from build123d import *

# Parameters (mm, degrees)
AUFSATZ_LINEAR_AUSTRAGEN1_DEPTH = 2.5


with BuildPart() as part:
    # Skizze1 → Rotation1 (revolve)
    with BuildSketch(Plane.XY):
        with BuildLine():
            Line((0, 45), (0, 35))
            ThreePointArc((0, 35), (5, 40), (0, 45))
        make_face()
    revolve(axis=Axis((0, 0, 0), (0, 1, 0)))

    # Skizze2 → Aufsatz-Linear austragen1 (add, symmetric)
    with BuildSketch(Plane.XY):
        Polygon((0, 40), (-10, 5.773502692), (0, 0), (10, 5.773502692), align=None)
    extrude(amount=AUFSATZ_LINEAR_AUSTRAGEN1_DEPTH, both=True)


solid = part.part
CAD build for the part. Positions are in the model's coordinates, mm. A direction names the side the tool comes from. Give positions to 0.01 mm unless a question says otherwise; leave off trailing zeros. Loops run counter-clockwise (first coordinate to the right, second up) from the corner with the lowest first, then second, coordinate; pieces in that order, holes last. Notation, with made-up numbers: M -37,53 L -10,53 A23 cw -10,81 Z; hole C -1.5,19.25 d10. An arc over 180 degrees is marked long. Write each question's results on one line, items separated by ' | '.
Q1. Mould opens along Y. For faces 3 (the face through (0, 14, -2.5)), 4 (the face through (5.67, 20.6, 0.04)), 5 (the face through (-5.07, 2.927, 0.035)) say: pulls with the +Y half, pulls with the -Y half, needs draft (parallel to the pull), parting line crosses it, or undercut.
Geometry check:
face 3: needs draft | face 4: undercut | face 5: pulls with the -Y half
Q2. Flat gauge pins, fed straight in: P1, Ø1.5, axis at y = 11, z = 1.5, coming from the +X side; P2, Ø4, axis at x = -0.5, y = 6, coming from the -Z side; P3, Ø4, axis at x = -6.5, z = 3.5, coming from the -Y side. Where does each tip first touch, or does it go through?
Geometry check:
P1: stops at x = 8.69 | P2: stops at z = -2.5 | P3: stops at y = 2.75
Q3. Band-saw the part on B-B on z = 3. Write the cut outline in (x, y), and give its area (3 significant figures).
Geometry check:
outline: C 0,40 d8 | area: 50.3 mm²
Q4. Which spindle directions (+Z, -Z, +X, -X, +Y, -Y) get a long thin tool onto all of the face, cutting with end or side? Do faces 1 (the face through (4.93, 2.846, 0.035)), 2 (the face through (0, 14, 2.5)). Say none if no direction does.
Geometry check:
face 1: +Z, -Z, +X, -Y | face 2: +Z, +X, -X, -Y
Q5. Band-saw the part on C-C on y = 27.5. Write the cut outline in (x, z).
Geometry check:
outline: M -3.65,-2.5 L 3.65,-2.5 L 3.65,2.5 L -3.65,2.5 Z
Q6. Band-saw the part on A-A on x = -3.25. Write the cut outline in (y, z).
Geometry check:
outline: M 1.88,-2.5 L 28.88,-2.5 L 28.88,2.5 L 1.88,2.5 Z; C 40,0 d7.6
Q7. Probe probe 1 along Z at (x, y) = (6.25, 13.5); probe 2 along Y at (x, z) = (0.75, -2); probe 3 along Y at (x, z) = (3.5, -3). List the from-to ranges inside material, lowest first.
Geometry check:
probe 1: z = -2.5 to 2.5 | probe 2: y = 0.43 to 44.52 | probe 3: y = 38.06 to 41.94
Q8. Band-saw the part on D-D on x = 3. Write the cut outline in (y, z), and give its area (3 significant figures).
Geometry check:
outline: M 1.73,-2.5 L 29.73,-2.5 L 29.73,2.5 L 1.73,2.5 Z; C 40,0 d8 | area: 190 mm²
